from build123d import *

# Parameters (mm, degrees)
ESBO_O1_R                = 45
RESSALTO_EXTRUS_O1_DEPTH = 10
CORTE_EXTRUS_O1_DEPTH    = 10
PADR_OCIRCULAR1_COUNT    = 4
ESBO_O3_R                = 3
RESSALTO_EXTRUS_O2_DEPTH = 8
RESSALTO_EXTRUS_O3_DEPTH = 8
PADR_OCIRCULAR2_COUNT    = 16


with BuildPart() as part:
    # Esboço1 → Ressalto-extrusão1 (new body)
    with BuildSketch(Plane.XY):
        Circle(ESBO_O1_R)
    extrude(amount=RESSALTO_EXTRUS_O1_DEPTH)

    # Esboço2 → Corte-extrusão1 (cut)
    with BuildSketch(Plane.XY.offset(10)):
        with BuildLine():
            Line((-19.67582712, 30.066816509), (-7.386402319, 13.055307763))
            ThreePointArc((-7.386402319, 13.055307763), (0, 15), (7.386402319, 13.055307763))
            Line((7.386402319, 13.055307763), (19.67582712, 30.066816509))
            ThreePointArc((19.67582712, 30.066816509), (0, 35.932598401), (-19.67582712, 30.066816509))
        make_face()
    corte_extrus_o1 = extrude(amount=-CORTE_EXTRUS_O1_DEPTH, mode=Mode.SUBTRACT)

    # PadrãoCircular1: Corte-extrusão1 ×4 about axis
    padr_ocircular1_axis = Axis((0, 0, 0), (0, 0, 1))
    for i in range(1, PADR_OCIRCULAR1_COUNT):
        add(corte_extrus_o1.rotate(padr_ocircular1_axis, i * 360 / PADR_OCIRCULAR1_COUNT), mode=Mode.SUBTRACT)

    # Esboço3 → Ressalto-extrusão2 (add)
    with BuildSketch(Plane.XY.offset(10)):
        Circle(ESBO_O3_R)
    extrude(amount=RESSALTO_EXTRUS_O2_DEPTH)

    # Esboço4 → Ressalto-extrusão3 (add)
    with BuildSketch(Plane.XY.offset(18)):
        Polygon((-0.5, 2.695095519), (0.5, 2.695095519), (0.314812798, 4.203324244), (-0.314812798, 4.203324244), align=None)
    ressalto_extrus_o3 = extrude(amount=-RESSALTO_EXTRUS_O3_DEPTH)

    # PadrãoCircular2: Ressalto-extrusão3 ×16 about axis
    padr_ocircular2_axis = Axis((0, 0, 0), (0, 0, 1))
    for i in range(1, PADR_OCIRCULAR2_COUNT):
        add(ressalto_extrus_o3.rotate(padr_ocircular2_axis, i * 360 / PADR_OCIRCULAR2_COUNT))


solid = part.part
Part model, mm, in its own coordinate system. Coordinates: 2 decimals unless noted, no trailing zeros. Order: outer loops, then holes, each group sorted by start corner. A loop starts at its lowest first (then second) coordinate and runs counter-clockwise, first axis right, second up.
(1) Probe L1, parallel to Y at x = 3.5, z = 16.75; L2, parallel to Y at x = 7.5, z = 9; L3, parallel to Z at x = -28.5, y = 19.5. List the from-to ranges inside material, lowest first.
Check sheet entries:
L1: y = -1.83 to -1.03, -0.4 to 0.4, 1.03 to 1.83
L2: y = -44.37 to -35.14, -13.21 to 13.21, 35.14 to 44.37
L3: z = 0 to 10
(2) Slice it at C-C, the plane y = -10.5. Write the cut outline in (x, z).
Check sheet entries:
outline: (-43.76, 0) - (-34.36, 0) - (-34.36, 10) - (-43.76, 10) - close; (-17.37, 0) - (17.37, 0) - (17.37, 10) - (-17.37, 10) - close; (34.36, 0) - (43.76, 0) - (43.76, 10) - (34.36, 10) - close
(3) Slice it at B-B, the plane x = 18.5. Write the cut outline in (y, z).
Check sheet entries:
outline: (-41.02, 0) - (-30.8, 0) - (-30.8, 10) - (-41.02, 10) - close; (-28.44, 0) - (-11.32, 0) - (-11.32, 10) - (-28.44, 10) - close; (11.32, 0) - (28.44, 0) - (28.44, 10) - (11.32, 10) - close; (30.8, 0) - (41.02, 0) - (41.02, 10) - (30.8, 10) - close
(4) Pin check, flat tips, straight feed: pin 1 Ø10 at (x, z) = (-1.5, 12.5) entering from +Y; pin 2 Ø0.7 at (x, z) = (0, 14.5) entering from -Y; pin 3 Ø1 at (x, z) = (33.5, 2.5) entering from +Y. Stop position of each tip, or through.
Check sheet entries:
pin 1: stops at y = 45
pin 2: stops at y = -4.2
pin 3: stops at y = 30.59
(5) Slice it at A-A, the plane z = 2.5. Write the cut outline in (x, y).
Check sheet entries:
outline: circle Ø90 at (0, 0); hole (-30.07, -19.68) - (-13.06, -7.39) arc R15 cw to (-13.06, 7.39) - (-30.07, 19.68) arc R35.93 ccw to start; hole (-19.68, -30.07) arc R35.93 ccw to (19.68, -30.07) - (7.39, -13.06) arc R15 cw to (-7.39, -13.06) - close; hole (-19.68, 30.07) - (-7.39, 13.06) arc R15 cw to (7.39, 13.06) - (19.68, 30.07) arc R35.93 ccw to start; hole (13.06, -7.39) - (30.07, -19.68) arc R35.93 ccw to (30.07, 19.68) - (13.06, 7.39) arc R15 cw to start
(6) Pull direction X, two halves, no side cores. Call faces 1 (the face through (20.765, -39.923, 4.93)), 2 (the face through (-21.442, 13.445, 5.07)), 3 (the face through (0, 0, 18)), 4 (the face through (0.29, 35.93, 5.07)): pulls with the +X half, pulls with the -X half, needs draft (parallel to the pull), parting line crosses it, or undercut.
Check sheet entries:
face 1: parting line crosses it
face 2: undercut
face 3: needs draft
face 4: undercut
(7) Slice it at D-D, the plane y = -23. Write the cut outline in (x, z), and give its area (3 significant figures).
Check sheet entries:
outline: (-38.68, 0) - (-14.57, 0) - (-14.57, 10) - (-38.68, 10) - close; (14.57, 0) - (38.68, 0) - (38.68, 10) - (14.57, 10) - close
area: 482 mm2
